Work out the finished part from the listing and answer in its coordinate system (mm). Coordinates: 2 decimals unless noted, no trailing zeros. Order: outer loops, then holes, each group sorted by start corner. A loop starts at its lowest first (then second) coordinate and runs counter-clockwise, first axis right, second up. Notation, with made-up numbers: M 74.25,7.25 L 115.25,7.25 A22 cw 115.25,17.25 Z; hole C 89.25,51 d2. An arc over 180 degrees is marked long. Use a Markdown table: item, result. Add a question column.
from build123d import *

# Parameters (mm, degrees)
F1_DEPTH = 69.85
F3_DEPTH = 9.525
F5_DEPTH = 9.525


with BuildPart() as f1:
    # F0 (on Front) → F1 (new body)
    with BuildSketch(Plane.XZ):
        Polygon((11.0363666468, 6.2839964384), (0.0760827704, 12.6997721008), (-10.9602838763, 6.4157756624), (-11.0363666468, -6.2839964384), (-0.0760827704, -12.6997721008), (10.9602838763, -6.4157756624), align=None)
    extrude(amount=F1_DEPTH)

    # F2 (on face) → F3 (cut)
    with BuildSketch(Plane.XZ.offset(69.85)):
        Polygon((-0.6350056975, 12.2948854617), (-0.6350056975, 0), (-0.6350056975, -12.372597718), (-0.0760827704, -12.6997721008), (0.634988605, -12.2948951939), (0.634988605, -0.0038041385), (0.634988605, 12.3726077233), (0.0760827704, 12.6997721008), align=None)
    extrude(amount=-F3_DEPTH, mode=Mode.SUBTRACT)

    # F4 (on face) → F5 (cut)
    with BuildSketch(Plane.XZ.offset(69.85)):
        with BuildLine():
            ThreePointArc((0.634988605, -1.9168625307), (1.6370407723, -1.1822309419), (2.0193, 0))
            ThreePointArc((2.0193, 0), (1.6370407723, 1.1822309419), (0.634988605, 1.9168625307))
            Line((0.634988605, 1.9168625307), (0.634988605, -1.9168625307))
        make_face()
        with BuildLine():
            Line((0.634988605, -1.9168625307), (0.634988605, 1.9168625307))
            ThreePointArc((0.634988605, 1.9168625307), (-2.0193, 0), (0.634988605, -1.9168625307))
        make_face()
    extrude(amount=-F5_DEPTH, mode=Mode.SUBTRACT)


solid = f1.part
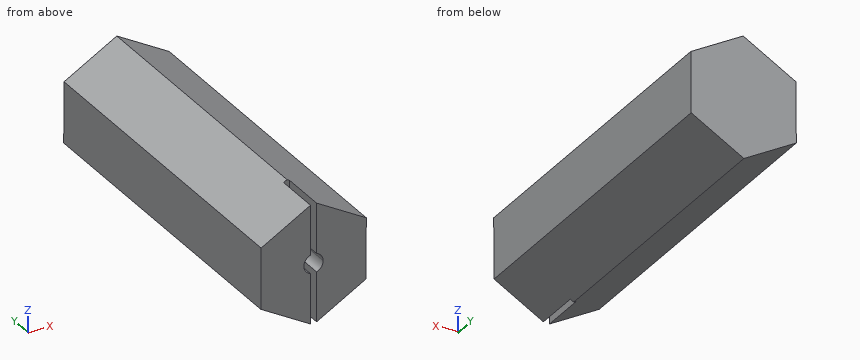
(1) A cutting plane is placed at B-B on z = 9.5. Write down the section's boundary in (x, y) (3 decimals).
(2) A cutting plane is placed at C-C on y = -31. Write down the section's boundary in (x, z).
(3) Straight lines are drawn through the part: line 1 (X direction, y = -34, z = 5.75); line 2 (Y direction, x = 0.5, z = 6.25) (3 decimals); line 3 (X direction, y = -62, z = -0.5). For each, find the intervals that lie inside material, in ascending order.
(4) Given P1, Ø7.5, axis at y = -67.5, z = 7, coming from the -X side; P2, Ø5, axis at x = -7, z = -3.5, coming from the +Y side; P3, Ø10.5, axis at y = -67, z = -9.5, coming from the +X side; P4, Ø6, axis at y = -15, z = 10, coming from the +X side, each flat-ended and moving along its own axis, determine where each tip first touches the part or whether it passes through.
(5) A cutting plane is placed at D-D on x = 6.75. Write down the section's boundary in (y, z).
(6) A cutting plane is placed at A-A on y = -63. Write down the section's boundary in (x, z) (3 decimals).
From the geometry:
| question | item | result |
|---|---|---|
| 1 | outline | M -5.544,-69.85 L -0.635,-69.85 L -0.635,-60.325 L 0.635,-60.325 L 0.635,-69.85 L 5.542,-69.85 L 5.542,0 L -5.544,0 Z |
| 2 | outline | M -11.04,-6.28 L -0.08,-12.7 L 10.96,-6.42 L 11.04,6.28 L 0.08,12.7 L -10.96,6.42 Z |
| 3 | line 1 | x = -10.96 to 11.03 |
| 3 | line 2 | y = -60.325 to 0 |
| 3 | line 3 | x = -11 to -1.96, 1.96 to 11 |
| 4 | P1 | stops at x = -10.98 |
| 4 | P2 | stops at y = 0 |
| 4 | P3 | stops at x = 10.97 |
| 4 | P4 | stops at x = 9.81 |
| 5 | outline | M -69.85,-8.81 L 0,-8.81 L 0,8.79 L -69.85,8.79 Z |
| 6 | outline | M -11.036,-6.284 L -0.635,-12.373 L -0.635,-1.917 A2.019 cw -0.635,1.917 L -0.635,12.295 L -10.96,6.416 Z; M 0.635,-12.295 L 10.96,-6.416 L 11.036,6.284 L 0.635,12.373 L 0.635,1.917 A2.019 cw 0.635,-1.917 Z |
